```python
from build123d import *

# Parameters (mm, degrees)
SKETCH2_R                        = 21.5
DISTANCE_HOLE_CUT_EXTRUDE1_DEPTH = 2


with BuildPart() as part:
    # Sketch1 → Chassi Revolve1 (revolve)
    with BuildSketch(Plane.XY):
        with BuildLine():
            Line((86.7, 68.7), (93.460307941, 2.2))
            Line((93.460307941, 2.2), (96.45, 2.2))
            ThreePointArc((96.45, 2.2), (97.65, 3.9), (98.85, 2.2))
            ThreePointArc((98.85, 2.2), (97.47607781, 0.687675162), (95.552047802, 0))
            Line((95.552047802, 0), (95.052047802, 0))
            ThreePointArc((95.052047802, 0), (92.953945214, 0.613594712), (91.45, 2.2))
            Line((91.45, 2.2), (85.574123323, 60))
            ThreePointArc((85.574123323, 60), (83.601573198, 62.573512221), (80.689692059, 64))
            Line((80.689692059, 64), (0, 64))
            Line((0, 64), (0, 66))
            Line((0, 66), (80.689692059, 66))
            ThreePointArc((80.689692059, 66), (83.110250345, 65.390210948), (85.169573298, 63.979489826))
            Line((85.169573298, 63.979489826), (84.689692059, 68.7))
            Line((84.689692059, 68.7), (86.7, 68.7))
        make_face()
    revolve(axis=Axis((0, 0, 0), (0, 1, 0)))

    # Sketch2 → Distance Hole Cut-Extrude1 (cut)
    with BuildSketch(Plane(origin=(0, 66, 0), x_dir=(1, 0, 0), z_dir=(0, 1, 0))):
        with Locations(Location((0, 0, 0), (0, 0, 180))):
            Circle(SKETCH2_R)
    extrude(amount=-DISTANCE_HOLE_CUT_EXTRUDE1_DEPTH, mode=Mode.SUBTRACT)


solid = part.part
```
The listing builds one solid part. Answer for the finished solid, in the listing's coordinates (mm). A direction names the side the tool comes from. Round coordinates to 2 decimals unless told otherwise and drop trailing zeros. Order: outer loops, then holes, each group sorted by start corner. A loop starts at its lowest first (then second) coordinate and runs counter-clockwise, first axis right, second up. Notation, with made-up numbers: (31.5, 57.25) - (79.5, 57.25) arc R11 cw to (79.5, 69.25) - close; hole circle Ø10 at (21.5, 12.25). An arc over 180 degrees is marked (long way). Put each result on its own line as item: value. Start each with the question number.
(1) Find section A-A (x = 0). Give the vertices of the cut face in (y, z).
(2) Find section D-D (y = 27.5). Give the vertices of the cut face in (x, z).
(3) Find section B-B (z = 0). Give the vertices of the cut face in (x, y).
(4) Determine the mould class of faces 1 (the flat face through (-19, 68.7, 83)), 2 (the conical face through (-19.04, 37.93, 85.73)) for opening direction Z: released by +Z, released by -Z, zero draft, split by the parting line, or undercut.
(5) Straight lines are drawn through the part: probe 1 along Z at (x, y) = (0, 64.75); probe 2 along Z at (x, y) = (0, 65.05); probe 3 along Y at (x, z) = (-9, -59). For each, find the intervals that lie inside material, in ascending order. Write a range as from..to.
(6) For faces 3 (the flat face through (-17, 66, 17)), 4 (the conical face through (-84.63, 68.47, -3.72)), 5 (the flat face through (17, 64, 17)), 6 (the cylindrical face through (2.799, 65.014, 21.317)), determine the directions among +Z, -Z, +X, -X, +Y, -Y from which every point of the face is accessible in a straight line to the end or side of a thin tool.
(7) Given P1, Ø2, axis at x = -59.5, z = -25.5, coming from the -Y side; P2, Ø3, axis at y = 40, z = -68.5, coming from the +X side; P3, Ø3, axis at x = 45, z = -31, coming from the +Y side, each flat-ended and moving along its own axis, determine where each tip first touches the part or whether it passes through.
(8) Find section C-C (y = 41.5). Give the vertices of the cut face in (x, z).
Reply:
1. outline: (0, -95.55) arc R4.21 ccw to (2.2, -98.85) arc R1.27 ccw (long way) to (2.2, -96.45) - (2.2, -93.46) - (68.7, -86.7) - (68.7, -84.69) - (63.98, -85.17) arc R7.09 ccw to (66, -80.69) - (66, -21.5) - (64, -21.5) - (64, -80.69) arc R7.09 cw to (60, -85.57) - (2.2, -91.45) arc R4.19 ccw to (0, -95.05) - close; (0, 95.05) arc R4.19 ccw to (2.2, 91.45) - (60, 85.57) arc R7.09 cw to (64, 80.69) - (64, 21.5) - (66, 21.5) - (66, 80.69) arc R7.09 ccw to (63.98, 85.17) - (68.7, 84.69) - (68.7, 86.7) - (2.2, 93.46) - (2.2, 96.45) arc R1.27 ccw (long way) to (2.2, 98.85) arc R4.21 ccw to (0, 95.55) - close
2. outline: circle Ø181.78 at (0, 0); hole circle Ø177.76 at (0, 0)
3. outline: (-98.85, 2.2) arc R4.21 ccw to (-95.55, 0) - (-95.05, 0) arc R4.19 ccw to (-91.45, 2.2) - (-85.57, 60) arc R7.09 cw to (-80.69, 64) - (-21.5, 64) - (-21.5, 66) - (-80.69, 66) arc R7.09 ccw to (-85.17, 63.98) - (-84.69, 68.7) - (-86.7, 68.7) - (-93.46, 2.2) - (-96.45, 2.2) arc R1.27 ccw (long way) to start; (21.5, 64) - (80.69, 64) arc R7.09 cw to (85.57, 60) - (91.45, 2.2) arc R4.19 ccw to (95.05, 0) - (95.55, 0) arc R4.21 ccw to (98.85, 2.2) arc R1.27 ccw (long way) to (96.45, 2.2) - (93.46, 2.2) - (86.7, 68.7) - (84.69, 68.7) - (85.17, 63.98) arc R7.09 ccw to (80.69, 66) - (21.5, 66) - close
4. face 1: zero draft
4. face 2: undercut
5. probe 1: -87.1..-85.09, -84.24..-21.5, 21.5..84.24, 85.09..87.1
5. probe 2: -87.07..-85.06, -83.77..-21.5, 21.5..83.77, 85.06..87.07
5. probe 3: 64..66
6. face 3: +Y
6. face 4: none
6. face 5: -Y
6. face 6: +Y, -Y
7. P1: y = 64
7. P2: x = 59.53
7. P3: y = 66
8. outline: circle Ø178.93 at (0, 0); hole circle Ø174.91 at (0, 0)
